```python
from build123d import *

# Parameters (mm, degrees)
SKETCH1_R                = 49
BOSS_EXTRUDE1_DEPTH      = 2.5
M3_CLEARANCE_HOLE1_D     = 3.6
M3_CLEARANCE_HOLE1_DEPTH = 20
M3_CLEARANCE_HOLE1_TIP   = 1.081549114
SKETCH4_R                = 31
CUT_EXTRUDE1_DEPTH       = 70.341545988
CHAMFER1_SIZE            = 0.3


with BuildPart() as part:
    # Sketch1 → Boss-Extrude1 (new body)
    with BuildSketch(Plane.XY):
        Circle(SKETCH1_R)
    extrude(amount=BOSS_EXTRUDE1_DEPTH)

    # M3 Clearance Hole1
    with Locations(Plane.XY.offset(2.5)):
        with Locations((-30.0520382, 30.0520382), (0, 42.5), (30.0520382, 30.0520382), (42.5, 0), (30.0520382, -30.0520382), (0, -42.5), (-30.0520382, -30.0520382), (-42.5, 0)):
            Hole(M3_CLEARANCE_HOLE1_D / 2, depth=M3_CLEARANCE_HOLE1_DEPTH)
            with Locations((0, 0, -(M3_CLEARANCE_HOLE1_DEPTH + M3_CLEARANCE_HOLE1_TIP / 2))):  # 118° drill point
                Cone(0, M3_CLEARANCE_HOLE1_D / 2, M3_CLEARANCE_HOLE1_TIP, mode=Mode.SUBTRACT)

    # Sketch4 → Cut-Extrude1 (cut, through all)
    with BuildSketch(Plane.XY.offset(2.5)):
        Circle(SKETCH4_R)
    extrude(amount=-CUT_EXTRUDE1_DEPTH, mode=Mode.SUBTRACT)

    # Chamfer1
    chamfer1_edges = [part.edges().sort_by_distance(p)[0] for p in [
        (-49, 0, 0),
        (-49, 0, 2.5),
        (-31, 0, 0),
        (-31, 0, 2.5),
    ]]
    chamfer(chamfer1_edges, length=CHAMFER1_SIZE)


solid = part.part
```
The model under review builds one solid part; all positions refer to its coordinate system, in mm. Round coordinates to 2 decimals unless told otherwise and drop trailing zeros. Loops run counter-clockwise (first coordinate to the right, second up) from the corner with the lowest first, then second, coordinate; pieces in that order, holes last. Notation, with made-up numbers: (22.25, 21.25) -> (81.25, 21.25) arc R29 ccw to (81.25, 45.25) -> close; hole circle Ø3 at (86.5, 33.5). An arc over 180 degrees is marked (long way). Answer in a Markdown table with one row per item.
1) For pin 1 Ø3 at (x, y) = (-30.05, 30.05) entering from +Z; pin 2 Ø4.5 at (x, y) = (-30.05, -30.05) entering from +Z; pin 3 Ø1 at (x, z) = (20.5, 0.5) entering from +Y, all flat-tipped, find the tip position at first contact; note any pin that passes through.
Taken from the geometry:
| item | result |
|---|---|
| pin 1 | passes through |
| pin 2 | stops at z = 2.5 |
| pin 3 | stops at y = 44.73 |
2) Consider section C-C, the plane z = 1.3. Count the separate pieces of the cut face and the enclosed holes in it, plus the area to 3 significant figures.
Taken from the geometry:
| item | result |
|---|---|
| separate pieces | 1 |
| enclosed holes | 9 |
| area | 4,440 mm² |
3) Wall thickness on line 1 along Y through (x, z) = (0, 1.7); line 2 along X through (y, z) = (1.5, 1.4); line 3 along X through (y, z) = (22, 2): over which ranges is each line inside the solid? List them lowest first.
Taken from the geometry:
| item | result |
|---|---|
| line 1 | y = -49 to -44.3, -40.7 to -31, 31 to 40.7, 44.3 to 49 |
| line 2 | x = -48.98 to -43.49, -41.51 to -30.96, 30.96 to 41.51, 43.49 to 48.98 |
| line 3 | x = -43.78 to -21.84, 21.84 to 43.78 |
4) Draft analysis for pull direction Y (two halves, no side actions). For faces 1 (the cylindrical face through (-4.036, 30.736, 1.263)), 2 (the flat face through (32, 1, 0)), 3 (the cylindrical face through (26.34, 41.32, 1.24)), state which applies: pulls with the +Y half, pulls with the -Y half, needs draft (parallel to the pull), parting line crosses it, or undercut.
Taken from the geometry:
| item | result |
|---|---|
| face 1 | undercut |
| face 2 | needs draft |
| face 3 | parting line crosses it |
5) Consider section A-A, the plane x = 0. Write out the cut boundary in (y, z), plus the area to 3 significant figures.
Taken from the geometry:
| item | result |
|---|---|
| outline | (-49, 0.3) -> (-48.7, 0) -> (-44.3, 0) -> (-44.3, 2.5) -> (-48.7, 2.5) -> (-49, 2.2) -> close; (-40.7, 0) -> (-31.3, 0) -> (-31, 0.3) -> (-31, 2.2) -> (-31.3, 2.5) -> (-40.7, 2.5) -> close; (31, 0.3) -> (31.3, 0) -> (40.7, 0) -> (40.7, 2.5) -> (31.3, 2.5) -> (31, 2.2) -> close; (44.3, 0) -> (48.7, 0) -> (49, 0.3) -> (49, 2.2) -> (48.7, 2.5) -> (44.3, 2.5) -> close |
| area | 71.6 mm² |
